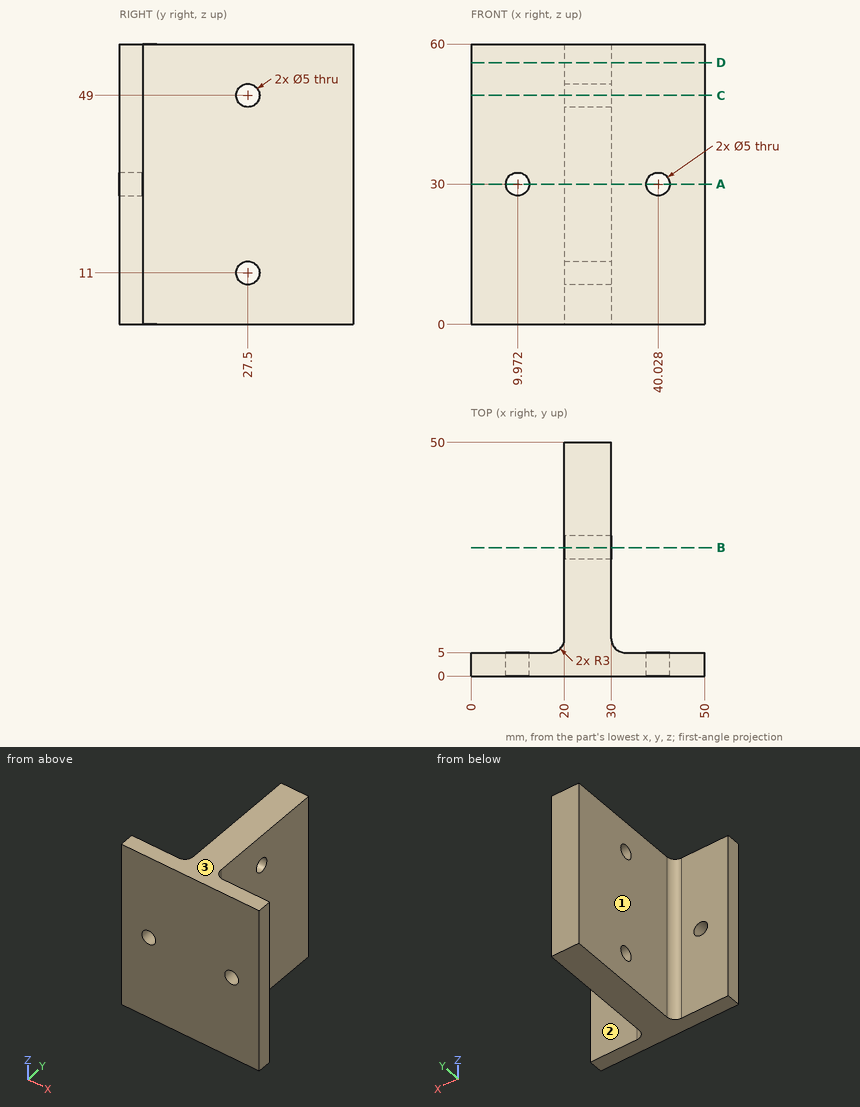
Drawing for the job (mm, zero at the part's lowest x, y, z). A direction names the side the tool comes from. Give positions to 0.01 mm unless a question says otherwise; leave off trailing zeros. Write each loop counter-clockwise with the first axis right and the second up, starting at its lowest first coordinate (ties: lowest second). Pieces come first, ordered by that corner, then holes. Notation, with made-up numbers: (-31.5, -34.75) -> (8.5, -34.75) arc R16 ccw to (8.5, -20.75) -> close; hole circle Ø11 at (50.25, -18). An arc over 180 degrees is marked (long way). Put each result on its own line as item: value. Start each with the question number.
Item 1: Cut at B-B (y = 27.5). List the corners of the cut face in (x, z).
Item 2: Cut at A-A (z = 30). List the corners of the cut face in (x, y).
Item 3: Which spindle directions (+Z, -Z, +X, -X, +Y, -Y) get a long thin tool onto all of the face, cutting with end or side? Do the marked faces 1, 2 and 3. Say none if no direction does.
Item 4: Pin check, flat tips, straight feed: pin 1 Ø6.5 at (x, z) = (9.97, 30) entering from +Y; pin 2 Ø8 at (x, y) = (19.5, 41.5) entering from +Z; pin 3 Ø21 at (y, z) = (21.5, 23.5) entering from +X; pin 4 Ø4.5 at (y, z) = (27.5, 11) entering from -X. Stop position of each tip, or through.
Item 5: Cut at D-D (z = 56). List the corners of the cut face in (x, y), then the cut area to 3 significant figures.
Item 6: Cut at C-C (z = 49). List the corners of the cut face in (x, y), then the cut area to 3 significant figures.
Item 7: Wall check: L1, parallel to X at y = 2, z = 30; L2, parallel to Y at x = 28, z = 11; L3, parallel to Z at x = 26, y = 27. Give the ranges that are in metal, low to high. Write a range as [from, to].
Answer list:
1. outline: (20, 0) -> (30, 0) -> (30, 8.5) -> (20, 8.5) -> close; (20, 13.5) -> (30, 13.5) -> (30, 46.5) -> (20, 46.5) -> close; (20, 51.5) -> (30, 51.5) -> (30, 60) -> (20, 60) -> close
2. outline: (0, 0) -> (7.47, 0) -> (7.47, 5) -> (0, 5) -> close; (12.47, 0) -> (37.53, 0) -> (37.53, 5) -> (33, 5) arc R3 cw to (30, 8) -> (30, 50) -> (20, 50) -> (20, 8) arc R3 cw to (17, 5) -> (12.47, 5) -> close; (42.53, 0) -> (50, 0) -> (50, 5) -> (42.53, 5) -> close
3. face 1: +Z, -Z, -X, +Y
3. face 2: +Z, -Z, +X, +Y
3. face 3: +Z, +X, -X, +Y, -Y
4. pin 1: stops at y = 5
4. pin 2: stops at z = 60
4. pin 3: stops at x = 30
4. pin 4: passes through
5. outline: (0, 0) -> (50, 0) -> (50, 5) -> (33, 5) arc R3 cw to (30, 8) -> (30, 50) -> (20, 50) -> (20, 8) arc R3 cw to (17, 5) -> (0, 5) -> close
5. area: 704 mm2
6. outline: (0, 0) -> (50, 0) -> (50, 5) -> (33, 5) arc R3 cw to (30, 8) -> (30, 25) -> (20, 25) -> (20, 8) arc R3 cw to (17, 5) -> (0, 5) -> close; (20, 30) -> (30, 30) -> (30, 50) -> (20, 50) -> close
6. area: 654 mm2
7. L1: x = [0, 7.47], [12.47, 37.53], [42.53, 50]
7. L2: y = [0, 25], [30, 50]
7. L3: z = [0, 8.55], [13.45, 46.55], [51.45, 60]
